The listing builds one solid part. Answer for the finished solid, in the listing's coordinates (mm). A direction names the side the tool comes from. Give positions to 0.01 mm unless a question says otherwise; leave off trailing zeros. Write each loop counter-clockwise with the first axis right and the second up, starting at its lowest first coordinate (ties: lowest second). Pieces come first, ordered by that corner, then holes. Notation, with made-up numbers: (84, 67) -> (110, 67) arc R12 cw to (110, 87) -> close; hole circle Ø3 at (1, -38.75). An arc over 180 degrees is marked (long way). One line per question, with ' | ' between items.
from build123d import *

# Parameters (mm, degrees)
BOSS_EXTRUDE1_DEPTH = 5
SKETCH2_W           = 5
SKETCH2_H           = 9.5
BOSS_EXTRUDE2_DEPTH = 1


with BuildPart() as part:
    # Sketch1 → Boss-Extrude1 (new body)
    with BuildSketch(Plane.XY):
        Polygon((0, 0), (0, 5), (5, 1.498962309), (5, -10), (0, -10), align=None)
    extrude(amount=BOSS_EXTRUDE1_DEPTH)

    # Sketch2 → Boss-Extrude2 (add)
    with BuildSketch(Plane.XZ.offset(10)):
        with Locations((2.5, 4.75)):
            Rectangle(SKETCH2_W, SKETCH2_H)
    extrude(amount=BOSS_EXTRUDE2_DEPTH)


solid = part.part
Item 1: Find section A-A (x = 0.5). Write down the section's boundary in (y, z), then the cut area to 3 significant figures.
Answers below:
outline: (-11, 0) -> (4.65, 0) -> (4.65, 5) -> (-10, 5) -> (-10, 9.5) -> (-11, 9.5) -> close | area: 82.7 mm²
Item 2: Consider line 1 (Y direction, x = 0.4, z = 5.25); line 2 (Z direction, x = 4, y = -3.5); line 3 (Y direction, x = 4.2, z = 1). Determine where each line is inside the solid, lowest interval first. Write a range as [from, to].
Answers below:
line 1: [-11, -10] | line 2: [0, 5] | line 3: [-11, 2.06]
Item 3: Find section D-D (x = 2.3). Write down the section's boundary in (y, z), then the cut area to 3 significant figures.
Answers below:
outline: (-11, 0) -> (3.39, 0) -> (3.39, 5) -> (-10, 5) -> (-10, 9.5) -> (-11, 9.5) -> close | area: 76.4 mm²
Item 4: Determine the mould class of faces 3 (the face through (3, -4, 5)), 4 (the face through (2, -3, 0)), 5 (the face through (0, -3, 3)) for opening direction Z: pulls with the +Z half, pulls with the -Z half, needs draft (parallel to the pull), parting line crosses it, or undercut.
Answers below:
face 3: pulls with the +Z half | face 4: pulls with the -Z half | face 5: needs draft
Item 5: Find section C-C (z = 6.75). Write down the section's boundary in (x, y).
Answers below:
outline: (0, -11) -> (5, -11) -> (5, -10) -> (0, -10) -> close
Item 6: A tool of negligible diameter and unlimited length cuts with its end or side. For faces 1 (the face through (2, -10, 7)), 2 (the face through (2, -11, 5)), from which of +Z, -Z, +X, -X, +Y, -Y can it reach the whole face along a straight path? Write none if from no direction.
Answers below:
face 1: +Z, +X, -X, +Y | face 2: +Z, -Z, +X, -X, -Y
Item 7: Find section B-B (y = -1.75). Write down the section's boundary in (x, z), then the cut area to 3 significant figures.
Answers below:
outline: (0, 0) -> (5, 0) -> (5, 5) -> (0, 5) -> close | area: 25.0 mm²
Item 8: Flat-ended cylindrical pins translate along their axes: pin 1 (1.5 mm diameter, centred on y = -8, z = 4, fed in from -X); pin 2 (1.5 mm diameter, centred on x = 2.5, y = 0, fed in from +Z); pin 3 (1.5 mm diameter, centred on x = 4, z = 8, fed in from +Y). Find the tip coordinate at first contact, or state that the pin passes through.
Answers below:
pin 1: x = 0 | pin 2: z = 5 | pin 3: y = -10
